For this review, take the finished solid that the model builds, in its own axes (mm). Face numbers are marked on the shaded views. Give positions to 0.01 mm unless a question says otherwise; leave off trailing zeros. Write each loop counter-clockwise with the first axis right and the second up, starting at its lowest first coordinate (ties: lowest second). Pieces come first, ordered by that corner, then holes.
Q1. We need section C-C (y = 5.1). Write out the cut boundary in (x, z), then the cut area to 3 significant figures.
Q2. Mouldability with a two-part tool opening along X and no side actions: class the marked faces 1, 2 and 3 as released by +X, released by -X, zero draft, split by the parting line, or undercut.
Q3. For line 1 (X direction, y = 3.1, z = 44.5); line 2 (Y direction, x = 4.5, z = 24); line 3 (Y direction, x = 9.25, z = 44), list the stretches that pass through material, from the lowest coordinate up.
Q4. We need section B-B (x = 2). Write out the cut boundary in (y, z), then the cut area to 3 significant figures.
Q5. We need section A-A (z = 40.5). Write out the cut boundary in (x, y).
Q6. Insertion check: P1, Ø5.5, axis at x = 5.5, z = 28.5, coming from the -Y side. The pin has a flat end and moves straight along its axis. Give the tip position at first contact, or say it passes through.
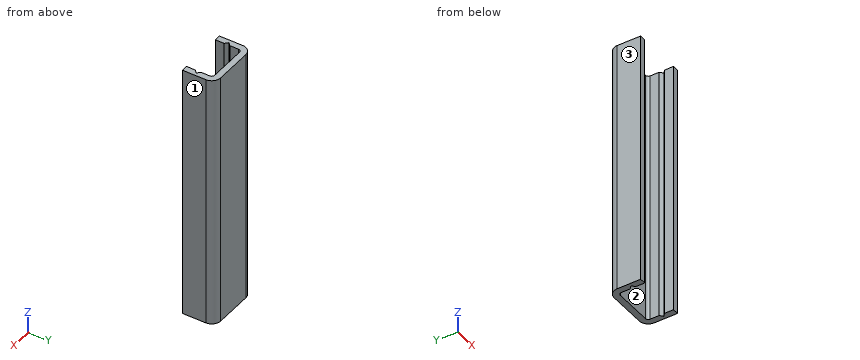
```python
from build123d import *

# Parameters (mm, degrees)
EXTRUSION1_DEPTH = 46


with BuildPart() as part:
    # Esquisse1 → Extrusion1 (new body)
    with BuildSketch(Plane.XY):
        with BuildLine():
            Line((1.6, 5.8), (8.4, 5.8))
            ThreePointArc((8.4, 5.8), (9.53137085, 5.33137085), (10, 4.2))
            Line((10, 4.2), (10, 0))
            Line((10, 0), (8.9, 0))
            Line((8.9, 0), (8.9, 1.6))
            Line((8.9, 1.6), (9.45, 2.1))
            Line((9.45, 2.1), (8.9, 2.6))
            Line((8.9, 2.6), (8.9, 4.2))
            ThreePointArc((8.9, 4.2), (8.753553391, 4.553553391), (8.4, 4.7))
            Line((8.4, 4.7), (1.6, 4.7))
            ThreePointArc((1.6, 4.7), (1.246446609, 4.553553391), (1.1, 4.2))
            Line((1.1, 4.2), (1.1, 2.6))
            Line((1.1, 2.6), (0.55, 2.1))
            Line((0.55, 2.1), (1.1, 1.6))
            Line((1.1, 1.6), (1.1, 0))
            Line((1.1, 0), (0, 0))
            Line((0, 0), (0, 4.2))
            ThreePointArc((0, 4.2), (0.46862915, 5.33137085), (1.6, 5.8))
        make_face()
    extrude(amount=EXTRUSION1_DEPTH)


solid = part.part
```
Computed:
1. outline: (0.28, 0) - (9.72, 0) - (9.72, 46) - (0.28, 46) - close
1. area: 435 mm2
2. face 1: released by +X
2. face 2: undercut
2. face 3: released by -X
3. line 1: x = 0 to 1.1, 8.9 to 10
3. line 2: y = 4.7 to 5.8
3. line 3: y = 0 to 1.92, 2.28 to 5.56
4. outline: (4.7, 0) - (5.8, 0) - (5.8, 46) - (4.7, 46) - close
4. area: 50.6 mm2
5. outline: (0, 0) - (1.1, 0) - (1.1, 1.6) - (0.55, 2.1) - (1.1, 2.6) - (1.1, 4.2) arc R0.5 cw to (1.6, 4.7) - (8.4, 4.7) arc R0.5 cw to (8.9, 4.2) - (8.9, 2.6) - (9.45, 2.1) - (8.9, 1.6) - (8.9, 0) - (10, 0) - (10, 4.2) arc R1.6 ccw to (8.4, 5.8) - (1.6, 5.8) arc R1.6 ccw to (0, 4.2) - close
6. P1: stops at y = 4.7
